Model file for the job. Use its own axes, mm. Face numbers are marked on the shaded views. Round coordinates to 2 decimals unless told otherwise and drop trailing zeros. Write each loop counter-clockwise with the first axis right and the second up, starting at its lowest first coordinate (ties: lowest second). Pieces come first, ordered by that corner, then holes.
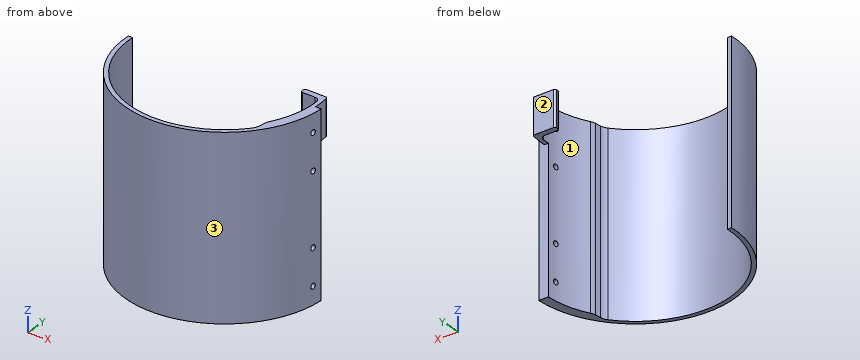
```python
from build123d import *

# Parameters (mm, degrees)
EXTRUDE_1_DEPTH     = 99.8
SKETCH_7_R          = 1.5
CUT_EXTRUDE_6_DEPTH = 80
CUT_EXTRUDE_7_DEPTH = 80


with BuildPart() as part:
    # 草图1 → 凸台-拉伸1 (new body)
    with BuildSketch(Plane.XY):
        with BuildLine():
            Line((-55, 0), (-52.6, 0))
            ThreePointArc((-52.6, 0), (-17.5838694, -49.573859411), (40.843632582, -33.144496941))
            ThreePointArc((40.843632582, -33.144496941), (41.8776275, -31.406850611), (42.371810697, -29.446150933))
            Line((42.371810697, -29.446150933), (42.701389329, -26.225087281))
            ThreePointArc((42.701389329, -26.225087281), (42.976584625, -24.872497257), (43.511842068, -23.600203386))
            ThreePointArc((43.511842068, -23.600203386), (48.437324754, -10.201743511), (49.33443696, 4.04516129))
            ThreePointArc((49.33443696, 4.04516129), (48.377266711, 6.006295976), (46.344471083, 6.8))
            Line((46.344471083, 6.8), (39, 6.8))
            ThreePointArc((39, 6.8), (38.292893219, 7.092893219), (38, 7.8))
            Line((38, 7.8), (38, 9))
            ThreePointArc((38, 9), (38.292893219, 9.707106781), (39, 10))
            Line((39, 10), (50.344019583, 10))
            ThreePointArc((50.344019583, 10), (50.805346897, 9.459374484), (51.0484918, 8.791557597))
            ThreePointArc((51.0484918, 8.791557597), (51.611780996, 4.411809423), (51.8, 0))
            Line((51.8, 0), (55, 0))
            ThreePointArc((55, 0), (0, -55), (-55, 0))
        make_face()
    extrude(amount=EXTRUDE_1_DEPTH)

    # 草图7 → 切除-拉伸6 (cut)
    with BuildSketch(Plane(origin=(0, 0, 0), x_dir=(0.10066073352284005, 0.994920809274107, 0), z_dir=(-0.9949208092741069, 0.10066073352284004, 0))):
        with Locations(Location((-0.136340344, -9.9, 0), (0, 0, 180))):
            Circle(SKETCH_7_R)
        with Locations(Location((-0.136340344, -29.9, 0), (0, 0, 180))):
            Circle(SKETCH_7_R)
        with Locations(Location((-0.136340344, -69.9, 0), (0, 0, 180))):
            Circle(SKETCH_7_R)
        with Locations(Location((-0.136340344, -89.9, 0), (0, 0, 180))):
            Circle(SKETCH_7_R)
    extrude(amount=-CUT_EXTRUDE_6_DEPTH, mode=Mode.SUBTRACT)

    # 草图8 → 切除-拉伸7 (cut)
    with BuildSketch(Plane(origin=(0, 0, 0), x_dir=(-1, 0, 0), z_dir=(0, 0, -1))):
        with BuildLine():
            Line((-50.016978469, 22.875792113), (0, 0))
            Line((0, 0), (-55, 0))
            ThreePointArc((-55, 0), (-53.739807479, 11.70611345), (-50.016978469, 22.875792113))
        make_face()
    extrude(amount=-CUT_EXTRUDE_7_DEPTH, mode=Mode.SUBTRACT)


solid = part.part
```
1) Wall check: probe 1 along X at (y, z) = (-27, 57); probe 2 along X at (y, z) = (-9, 8.5); probe 3 along Y at (x, z) = (0.5, 36). Give the ranges that are in metal, low to high.
2) Cut at B-B on y = -48.5. List the corners of the cut face in (x, z), and give its area (3 significant figures).
3) Pull direction X, two halves, no side cores. Call the marked faces 1, 2 and 3: released by +X, released by -X, zero draft, split by the parting line, or undercut.
4) Cut at C-C on x = 0. List the corners of the cut face in (y, z).
5) Cut at A-A on z = 36. List the corners of the cut face in (x, y).
6) Cut at D-D on y = 1.5. List the corners of the cut face in (x, z).
7) Flat gauge pins, fed straight in: pin 1 Ø2 at (y, z) = (-35.5, 41) entering from -X; pin 2 Ø6 at (x, z) = (19.5, 31.5) entering from +Y; pin 3 Ø8 at (x, z) = (13, 24) entering from +Y. Where does each tip first touch, or does it go through?
Result sheet:
1. probe 1: x = -47.92 to -45.14, 42.62 to 47.92
1. probe 2: x = -54.26 to -51.82, 48.67 to 54.26
1. probe 3: y = -55 to -52.6
2. outline: (-25.94, 0) - (-20.36, 0) - (-20.36, 99.8) - (-25.94, 99.8) - close; (20.36, 0) - (25.94, 0) - (25.94, 99.8) - (20.36, 99.8) - close
2. area: 1,110 mm2
3. face 1: undercut
3. face 2: zero draft
3. face 3: split by the parting line
4. outline: (-55, 0) - (-52.6, 0) - (-52.6, 99.8) - (-55, 99.8) - close
5. outline: (-55, 0) arc R55 ccw to (55, 0) - (49.5, 0) arc R49.5 cw to (43.51, -23.6) arc R7 ccw to (42.7, -26.23) - (42.37, -29.45) arc R7 cw to (40.84, -33.14) arc R52.6 cw to (-52.6, 0) - close
6. outline: (49.48, 80) - (51.78, 80) - (51.78, 99.8) - (49.48, 99.8) - close
7. pin 1: stops at x = -42.83
7. pin 2: stops at y = -47.54
7. pin 3: stops at y = -49.78
